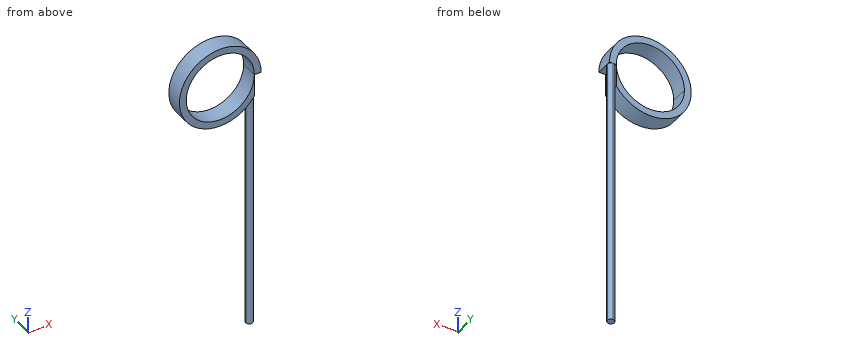
Autodesk Inventor part; units mm, degrees
ref_plane "YZ Plane" through (0, 0, 0) normal (1, 0, 0) x (0, 1, 0)
ref_plane "XZ Plane" through (0, 0, 0) normal (0, 1, 0) x (-1, 0, 0)
ref_plane "XY Plane" through (0, 0, 0) normal (0, 0, 1) x (1, 0, 0)
sketch "スケッチ1" plane through (0, 0, 0) normal (0, 1, 0) x (-1, 0, 0)
  circle A0 centre (0, 0) radius 2.5
  circle A1 centre (0, 0) radius 3
  line L0 (-2.5, 0) -> (-3, 0)
  line L1 (-3, 0) -> (-3, -20)
  line L2 (-3, -20) -> (-2.5, -20)
  line L3 (-2.5, -20) -> (-2.5, 0)
  point P0 (-2.5, -1.6583)
  dimension "d0" = 5
  dimension "d1" = 6
  dimension "d2" = 20
extrude "押し出し1" add sketch "スケッチ1" along normal blind 1.25
sketch "スケッチ2" plane through (3, 0, -20) normal (0, 0, -1) x (-1, 0, 0)
  line L0 (0, 0) -> (0.5, 0)
  line L1 (0.5, 0) -> (0.5, 1.25)
  line L2 (0, 1.25) -> (0.5, 1.25)
  line L3 (0, 0) -> (0, 1.25)
  circle A0 centre (0.25, 1) radius 0.25
  line L4 (0, 1.25) -> (0.5, 1.25)
  line L5 (0.5, 0) -> (0.5, 1.25)
  point P0 (3, 0)
  point P1 (0, 1)
  point P2 (0.25, 1.25)
  point P3 (0.5, 1)
extrude "押し出し2" cut sketch "スケッチ2" against normal blind 20 contours L3 A0 L1 L0 | L3 L2 A0 | A0 L2 L1
properties part number "spring_180(131)" material "アルミニウム 6061"
The model under review builds one solid part; all positions refer to its coordinate system, in mm. Coordinates: 2 decimals unless noted, no trailing zeros. Write each loop counter-clockwise with the first axis right and the second up, starting at its lowest first coordinate (ties: lowest second). Pieces come first, ordered by that corner, then holes. Notation, with made-up numbers: (49.25, 75) - (59.25, 75) arc R32 ccw to (59.25, 111) - close; hole circle Ø8 at (57, -5). An arc over 180 degrees is marked (long way). Answer in a Markdown table with one row per item. Add a question column.
Q1. To check wall thickness, follow line 1 along Z through (x, y) = (-1.25, 0.6); line 2 along X through (y, z) = (1, -16.5); line 3 along Z through (x, y) = (-2, 0.35). State the ranges of each line that lie inside material, in increasing order. Write a range as from..to.
Q2. Consider section C-C on x = 1.25. Give the boundary of the cut face in (y, z).
Q3. Consider section A-A on x = 0. Give the boundary of the cut face in (y, z).
Q4. Consider section D-D on z = -13.5. Give the boundary of the cut face in (x, y).
Answers below:
| question | item | result |
|---|---|---|
| 1 | line 1 | -2.73..-2.17, 2.17..2.73 |
| 1 | line 2 | 2.5..3 |
| 1 | line 3 | -2.24..-1.5, 1.5..2.24 |
| 2 | outline | (0, -2.73) - (1.25, -2.73) - (1.25, -2.17) - (0, -2.17) - close; (0, 2.17) - (1.25, 2.17) - (1.25, 2.73) - (0, 2.73) - close |
| 3 | outline | (0, -3) - (1.25, -3) - (1.25, -2.5) - (0, -2.5) - close; (0, 2.5) - (1.25, 2.5) - (1.25, 3) - (0, 3) - close |
| 4 | outline | circle Ø0.5 at (2.75, 1) |
